Input: part model. Units: mm. Frame: model coordinates. A direction names the side the tool comes from. Coordinates: 2 decimals unless noted, no trailing zeros. Order: outer loops, then holes, each group sorted by start corner. A loop starts at its lowest first (then second) coordinate and runs counter-clockwise, first axis right, second up. Notation, with made-up numbers: (36, 77.25) -> (78, 77.25) arc R33 cw to (78, 116.25) -> close; hole circle Ø11 at (37, -17). An arc over 180 degrees is marked (long way). Use CSV: the item, a comma, the result in double quotes. Start each with the question number.
```python
from build123d import *

# Parameters (mm, degrees)
F1_DEPTH  = 42.5
F2_W      = 3
F2_H      = 70
F2_W_2    = 65.5
F3_DEPTH  = 9
F3_FACE_W = 71.5
F3_FACE_H = 85
F4_DEPTH  = 3


with BuildPart() as f1:
    # F0 (on Front) → F1 (new body, symmetric)
    with BuildSketch(Plane.XZ):
        Polygon((22.3621103702, 109.2680796906), (-8.3229273872, 30), (0, 26.5752547967), (28.090155991, 99.1349922478), (30.7552011609, 106.0190756927), align=None)
        with BuildLine():
            Line((28.090155991, 99.1349922478), (0, 26.5752547967))
            Line((0, 26.5752547967), (12.916813397, 21.2602024521))
            Line((12.916813397, 21.2602024521), (29.2348995336, 98.7953817902))
            ThreePointArc((29.2348995336, 98.7953817902), (28.6556498353, 98.9420032142), (28.090155991, 99.1349922478))
        make_face()
        with BuildLine():
            Line((30.3524578973, 98.6481280943), (30.7552011609, 106.0190756927))
            Line((30.7552011609, 106.0190756927), (29.2348995336, 98.7953817902))
            ThreePointArc((29.2348995336, 98.7953817902), (29.7908639139, 98.7003924567), (30.3524578973, 98.6481280943))
        make_face()
        with BuildLine():
            Line((31.3717730218, 98.662927939), (30.7552011609, 106.0190756927))
            Line((30.7552011609, 106.0190756927), (30.3524578973, 98.6481280943))
            ThreePointArc((30.3524578973, 98.6481280943), (30.8623712412, 98.637911475), (31.3717730218, 98.662927939))
        make_face()
        with BuildLine():
            Line((30.7552011609, 106.0190756927), (28.090155991, 99.1349922478))
            ThreePointArc((28.090155991, 99.1349922478), (28.6556498353, 98.9420032142), (29.2348995336, 98.7953817902))
            Line((29.2348995336, 98.7953817902), (30.7552011609, 106.0190756927))
        make_face()
        with BuildLine():
            Line((32.2561050406, 98.7913265148), (30.7552011609, 106.0190756927))
            Line((30.7552011609, 106.0190756927), (31.3717730218, 98.662927939))
            ThreePointArc((31.3717730218, 98.662927939), (31.8158836896, 98.713733592), (32.2561050406, 98.7913265148))
        make_face()
        with BuildLine():
            ThreePointArc((32.2561050406, 98.7913265148), (32.6301854549, 98.8792224357), (32.9991851562, 98.9864654757))
            Line((32.9991851562, 98.9864654757), (30.7552011609, 106.0190756927))
            Line((30.7552011609, 106.0190756927), (32.2561050406, 98.7913265148))
        make_face()
        with BuildLine():
            Line((25.8336267941, 15.9451501074), (38.7504401911, 10.6300977628))
            Line((38.7504401911, 10.6300977628), (31.3717730218, 98.662927939))
            ThreePointArc((31.3717730218, 98.662927939), (30.8623712412, 98.637911475), (30.3524578973, 98.6481280943))
            Line((30.3524578973, 98.6481280943), (25.8336267941, 15.9451501074))
        make_face()
        with BuildLine():
            Line((51.6672535881, 5.3150454182), (64.5840501522, 0))
            Line((64.5840501522, 0), (32.9991851562, 98.9864654757))
            ThreePointArc((32.9991851562, 98.9864654757), (32.6301854549, 98.8792224357), (32.2561050406, 98.7913265148))
            Line((32.2561050406, 98.7913265148), (51.6672535881, 5.3150454182))
        make_face()
        Polygon((-8.3229273872, 30), (-20.4159498478, 0), (64.5840501522, 0), (51.6672535881, 5.3150454182), (38.7504401911, 10.6300977628), (25.8336267941, 15.9451501074), (12.916813397, 21.2602024521), (0, 26.5752547967), align=None)
    extrude(amount=F1_DEPTH, both=True)

    # F2 (on face) → F3 (cut)
    with BuildSketch(Plane(origin=(-17.3379708436, 0, 6.7116081536), x_dir=(0, -1, 0), z_dir=(-0.9325656434, 0, 0.3610004442))):
        with Locations((34.1458392143, 74.9723888187)):
            Rectangle(F2_W, F2_H)
        with Locations((-0.1041607857, 74.9723888187)):
            Rectangle(F2_W_2, F2_H)
        with Locations((-34.3541607857, 74.9723888187)):
            Rectangle(F2_W, F2_H)
        Polygon((-35.8541607857, 35.0806618999), (-35.8541607857, 24.9723888187), (-32.8541607857, 24.9723888187), (-32.8541607857, 39.9723888187), (-35.8541607857, 39.9723888187), align=None)
        Polygon((-32.8541607857, 39.9723888187), (-32.8541607857, 24.9723888187), (-0.1041607857, 24.9723888187), (32.6458392143, 24.9723888187), (32.6458392143, 39.9723888187), align=None)
        Polygon((32.6458392143, 39.9723888187), (32.6458392143, 24.9723888187), (35.6458392143, 24.9723888187), (35.6458392143, 35.0806618999), (35.6458392143, 39.9723888187), align=None)
    extrude(amount=-F3_DEPTH, mode=Mode.SUBTRACT)

    # F3_face (on face) + F2 (on face) + F1_face1 (on face) → F4 (join)
    with BuildSketch(Plane(origin=(15.4126822823, 0.1041607857, 66.3850358474), x_dir=(0, -1, 0), z_dir=(-0.9325656434, 0, 0.3610004442))):
        Rectangle(F3_FACE_W, F3_FACE_H)
    with BuildSketch(Plane(origin=(-17.3379708436, 0, 6.7116081536), x_dir=(0, -1, 0), z_dir=(-0.9325656434, 0, 0.3610004442))):
        with Locations((-34.3541607857, 74.9723888187)):
            Rectangle(F2_W, F2_H)
        Polygon((-35.8541607857, 35.0806618999), (-35.8541607857, 24.9723888187), (-32.8541607857, 24.9723888187), (-32.8541607857, 39.9723888187), (-35.8541607857, 39.9723888187), align=None)
        Polygon((-32.8541607857, 39.9723888187), (-32.8541607857, 24.9723888187), (-0.1041607857, 24.9723888187), (32.6458392143, 24.9723888187), (32.6458392143, 39.9723888187), align=None)
        Polygon((32.6458392143, 39.9723888187), (32.6458392143, 24.9723888187), (35.6458392143, 24.9723888187), (35.6458392143, 35.0806618999), (35.6458392143, 39.9723888187), align=None)
        with Locations((34.1458392143, 74.9723888187)):
            Rectangle(F2_W, F2_H)
        Polygon((-42.5, 24.9723888187), (-35.8541607857, 24.9723888187), (-35.8541607857, 35.0806618999), (-35.8541607857, 39.9723888187), (-35.8541607857, 109.9723888187), (-42.5, 109.9723888187), align=None)
        Polygon((35.6458392143, 35.0806618999), (35.6458392143, 24.9723888187), (42.5, 24.9723888187), (42.5, 109.9723888187), (35.6458392143, 109.9723888187), (35.6458392143, 39.9723888187), align=None)
    with BuildSketch(Plane(origin=(-14.3694386175, 0, 15), x_dir=(0, -1, 0), z_dir=(-0.9274816955, 0, 0.3738685658))):
        Polygon((-35.8541607857, 16.1728259144), (-42.5, 16.1728259144), (-42.5, -16.1728259144), (42.5, -16.1728259144), (42.5, 16.1728259144), (35.6458392143, 16.1728259144), align=None)
    extrude(amount=F4_DEPTH, dir=(-0.9325656434, 0, 0.3610004442))


solid = f1.part
```
1. Contact query for flat-ended pins moving along their axis: P1, Ø6, axis at y = 8, z = 23.5, coming from the -X side; P2, Ø4, axis at y = -30, z = 44.5, coming from the -X side; P3, Ø3, axis at x = 27, z = 43.5, coming from the -Y side; P4, Ø10, axis at y = -28, z = 62.5, coming from the +X side. Output: stop coordinate, or through.
2. Section D-D on z = 42. Return loops of the section in (x, y).
3. Material intervals for line 1 along X through (y, z) = (-30.5, 97); line 2 along X through (y, z) = (-18, 73); line 3 along X through (y, z) = (3, 41.5), sorted ascending.
4. Section C-C on x = 45. Return loops of the section in (y, z).
5. Access query for faces 4 (the face through (10, -35.646, 68)), 5 (the face through (19.466, -0.595, 18.565)), 6 (the face through (-4.287, -0.354, 44.522)). Directions: +Z, -Z, +X, -X, +Y, -Y. A direction counts if a zero-diameter tool reaches every point of the face in a straight line with its end or side. Return the directions, or none.
6. Section A-A on y = 23. Return loops of the section in (x, z).
7. Pull-direction query (X, two-part tool) for faces 1 (the face through (21, -1, 0)), 2 (the face through (41.826, -0.595, 52.708)), 3 (the face through (-5.79, 0.59, 44.85)); classes: released by +X, released by -X, zero draft, split by the parting line, or undercut.
8. Section B-B on z = 83. Return loops of the section in (x, y).
Values follow:
1,P1,"stops at x = -15.39"
1,P2,"stops at x = -6.7"
1,P3,"stops at y = -42.5"
1,P4,"stops at x = 46.24"
2,outline,"(-6.89, -42.5) -> (17.28, -42.5) -> (17.28, 42.5) -> (-6.89, 42.5) -> close; (27.26, -42.5) -> (36.12, -42.5) -> (36.12, 42.5) -> (27.26, 42.5) -> close; (44.05, -42.5) -> (51.18, -42.5) -> (51.18, 42.5) -> (44.05, 42.5) -> close; hole (-3.68, -35.65) -> (2.76, -35.65) -> (2.76, 35.85) -> (-3.68, 35.85) -> close"
3,line 1,"x = 24.05 to 28.86, 30.26 to 31.51, 32.63 to 33.63"
3,line 2,"x = 14.76 to 23.81, 28.95 to 33.52, 37.61 to 41.29"
3,line 3,"x = -7.09 to -3.87, 2.56 to 17.18, 27.23 to 36.16, 44.15 to 51.34"
4,outline,"(-42.5, 0) -> (42.5, 0) -> (42.5, 8.06) -> (-42.5, 8.06) -> close; (-42.5, 37.42) -> (42.5, 37.42) -> (42.5, 61.38) -> (-42.5, 61.38) -> close"
5,face 4,"none"
5,face 5,"+Y, -Y"
5,face 6,"+Z"
6,outline,"(-23.21, 1.08) -> (-20.42, 0) -> (64.58, 0) -> (30.76, 106.02) -> (27.96, 107.1) -> (-2.73, 27.83) -> (-8.32, 30) -> (-2.91, 43.99) -> (-5.71, 45.07) -> (-11.12, 31.08) -> close; hole (12.92, 21.26) -> (25.83, 15.95) -> (30.35, 98.65) arc R7.38 cw to (29.23, 98.8) -> close; hole (31.37, 98.66) -> (38.75, 10.63) -> (51.67, 5.32) -> (32.26, 98.79) arc R7.38 cw to start"
7,face 1,"zero draft"
7,face 2,"undercut"
7,face 3,"released by -X"
8,outline,"(8.98, -42.5) -> (25.91, -42.5) -> (25.91, 42.5) -> (8.98, 42.5) -> (8.98, 32.85) -> (12.19, 32.85) -> (12.19, 35.85) -> (18.63, 35.85) -> (18.63, -35.65) -> (12.19, -35.65) -> (12.19, -32.65) -> (8.98, -32.65) -> close; (29.5, -42.5) -> (32.68, -42.5) -> (32.68, 42.5) -> (29.5, 42.5) -> close; (35.54, -42.5) -> (38.1, -42.5) -> (38.1, 42.5) -> (35.54, 42.5) -> close"
